from build123d import *

# Parameters (mm, degrees)
BOSS_EXTRUDE1_DEPTH = 6
BOSS_EXTRUDE2_DEPTH = 3
SKETCH3_W           = 15
SKETCH3_H           = 14.578547678
CUT_EXTRUDE1_DEPTH  = 3
CUT_EXTRUDE2_DEPTH  = 0.1
FILLET1_R           = 3
CHAMFER1_SIZE       = 0.528980942
CHAMFER1_SIZE_2     = 3


with BuildPart() as part:
    # Sketch1 → Boss-Extrude1 (new body)
    with BuildSketch(Plane(origin=(0, 0, 0), x_dir=(1, 0, 0), z_dir=(0, 1, 0))):
        with BuildLine():
            Line((22.5, -167.846096908), (22.5, -150.861139315))
            ThreePointArc((22.5, -150.861139315), (0, -153.564064606), (-22.5, -150.861139315))
            Line((-22.5, -150.861139315), (-22.5, -167.846096908))
            Line((-22.5, -167.846096908), (22.5, -167.846096908))
        make_face()
        with BuildLine():
            Line((-17.5, -154.846096908), (-17.5, -160.846096908))
            ThreePointArc((-17.5, -160.846096908), (-15.75, -162.596096908), (-14, -160.846096908))
            Line((-14, -160.846096908), (-14, -154.846096908))
            ThreePointArc((-14, -154.846096908), (-15.75, -153.096096908), (-17.5, -154.846096908))
        make_face(mode=Mode.SUBTRACT)
        with BuildLine():
            Line((14, -154.846096908), (14, -160.846096908))
            ThreePointArc((14, -160.846096908), (15.75, -162.596096908), (17.5, -160.846096908))
            Line((17.5, -160.846096908), (17.5, -154.846096908))
            ThreePointArc((17.5, -154.846096908), (15.75, -153.096096908), (14, -154.846096908))
        make_face(mode=Mode.SUBTRACT)
    extrude(amount=BOSS_EXTRUDE1_DEPTH)

    # Sketch2 → Boss-Extrude2 (add)
    with BuildSketch(Plane(origin=(0, 0, 0), x_dir=(1, 0, 0), z_dir=(0, 1, 0))):
        with BuildLine():
            Line((-22.5, -167.846096908), (22.5, -167.846096908))
            Line((22.5, -167.846096908), (22.5, -150.861139315))
            Line((22.5, -150.861139315), (10.691043752, -131.369092702))
            ThreePointArc((10.691043752, -131.369092702), (0, -125.346096908), (-10.691043752, -131.369092702))
            Line((-10.691043752, -131.369092702), (-22.5, -150.861139315))
            Line((-22.5, -150.861139315), (-22.5, -167.846096908))
        make_face()
        with BuildLine():
            Line((-17.5, -154.846096908), (-17.5, -160.846096908))
            ThreePointArc((-17.5, -160.846096908), (-15.75, -162.596096908), (-14, -160.846096908))
            Line((-14, -160.846096908), (-14, -154.846096908))
            ThreePointArc((-14, -154.846096908), (-15.75, -153.096096908), (-17.5, -154.846096908))
        make_face(mode=Mode.SUBTRACT)
        with BuildLine():
            Line((14, -154.846096908), (14, -160.846096908))
            ThreePointArc((14, -160.846096908), (15.75, -162.596096908), (17.5, -160.846096908))
            Line((17.5, -160.846096908), (17.5, -154.846096908))
            ThreePointArc((17.5, -154.846096908), (15.75, -153.096096908), (14, -154.846096908))
        make_face(mode=Mode.SUBTRACT)
    extrude(amount=BOSS_EXTRUDE2_DEPTH)

    # Sketch3 → Cut-Extrude1 (cut)
    with BuildSketch(Plane(origin=(0, 6, 0), x_dir=(1, 0, 0), z_dir=(0, 1, 0))):
        with Locations((0, -160.556823069)):
            Rectangle(SKETCH3_W, SKETCH3_H)
    extrude(amount=-CUT_EXTRUDE1_DEPTH, mode=Mode.SUBTRACT)

    # Sketch4 → Cut-Extrude2 (cut)
    with BuildSketch(Plane(origin=(0, 3, 0), x_dir=(1, 0, 0), z_dir=(0, 1, 0))):
        with BuildLine():
            Line((-4.25, -146.342419642), (-4.25, -167.846096908))
            Line((-4.25, -167.846096908), (4.25, -167.846096908))
            Line((4.25, -167.846096908), (4.25, -146.342419642))
            ThreePointArc((4.25, -146.342419642), (0, -128.346096908), (-4.25, -146.342419642))
        make_face()
    extrude(amount=-CUT_EXTRUDE2_DEPTH, mode=Mode.SUBTRACT)

    # Fillet1
    # the kernel refuses this fillet: 3 mm, written as the material it takes off along each edge
    with BuildSketch(Plane(origin=(-4.25, 2.9, 167.846096908), x_dir=(0, -1, 0), z_dir=(1, 0, 0))) as fillet1_piece_1:
        with BuildLine():
            CenterArc((FILLET1_R, FILLET1_R), FILLET1_R, 180, 90)
            Line((0, FILLET1_R), (0, 0))
            Line((0, 0), (FILLET1_R, 0))
        make_face()
    extrude(amount=8.5, mode=Mode.SUBTRACT)

    # Chamfer1
    # the kernel refuses this chamfer: 3, 0.528980942 mm, written as the material it takes off along each edge
    with BuildSketch(Plane(origin=(26.539379212, 3, 157.528601387), x_dir=(0.1797282148286355, -0.9776715712462603, -0.10888557099717337), z_dir=(-0.5181603365296565, 0, -0.8552835001608959))) as chamfer1_piece_1_section:
        Polygon((CHAMFER1_SIZE * 0.977671571478, CHAMFER1_SIZE * 0.210138760817), (-CHAMFER1_SIZE_2 * 0.210138760767, CHAMFER1_SIZE_2 * 0.977671571246), (0, 0), align=None)
    chamfer1_piece_1 = extrude(amount=30.585774986, mode=Mode.PRIVATE)
    chamfer1_piece_1 = chamfer1_piece_1 & Plane(origin=(0, 2.81678549, 58.564064606), x_dir=(0.23684210526315766, 0, 0.9715481548407755), z_dir=(0, -1, 0)) * Cylinder(95, 73, mode=Mode.PRIVATE)
    add(chamfer1_piece_1, mode=Mode.SUBTRACT)
    with BuildSketch(Plane(origin=(0, 3, 137.846096908), x_dir=(0.8552835001609747, 0, -0.5181603365295261), z_dir=(0.5181603365295261, 0, 0.8552835001609747))) as chamfer1_piece_2:
        Polygon((12.5, -CHAMFER1_SIZE), (12.5 - CHAMFER1_SIZE_2, 0), (12.5, 0), align=None)
    revolve(axis=Axis((0, 3, 137.846096908), (0, 1, 0)), revolution_arc=117.582137566, mode=Mode.SUBTRACT)
    with BuildSketch(Plane(origin=(-10.691043752, 3, 131.369092702), x_dir=(0.8552644030796279, 0.0066825316561016845, 0.5181487668570801), z_dir=(-0.5181603365296562, 0, 0.855283500160896))) as chamfer1_piece_3_section:
        Polygon((CHAMFER1_SIZE_2 * 0.999977671636, -CHAMFER1_SIZE_2 * 0.0066825316561), (-CHAMFER1_SIZE * 0.00668253165769, -CHAMFER1_SIZE * 0.999977671873), (0, 0), align=None)
    chamfer1_piece_3 = extrude(amount=30.585774986, mode=Mode.PRIVATE)
    chamfer1_piece_3 = chamfer1_piece_3 & Plane(origin=(0, 2.847950314, 58.564064606), x_dir=(0.23684210526315766, 0, 0.9715481548407755), z_dir=(0, -1, 0)) * Cylinder(95, 74, mode=Mode.PRIVATE)
    add(chamfer1_piece_3, mode=Mode.SUBTRACT)


solid = part.part
Verification items for the finished model (mm, model axes). A direction names the side the tool comes from. Give positions to 0.01 mm unless a question says otherwise; leave off trailing zeros. Write each loop counter-clockwise with the first axis right and the second up, starting at its lowest first coordinate (ties: lowest second). Pieces come first, ordered by that corner, then holes.
(1) Gauge pin test, flat ends, axial feed: pin 1 (1.5 mm diameter, centred on y = 2.5, z = 131, fed in from -X); pin 2 (8 mm diameter, centred on x = -3, z = 149.5, fed in from +Y); pin 3 (1 mm diameter, centred on y = 2, z = 137, fed in from -X). Record the tip position at first contact, or that the pin passes through.
(2) Cross-section at D-D (y = 0.9). Enter the section's corners in (x, z), plus the area to 3 significant figures.
(3) Material ranges on line 1 (X direction, y = 1.7, z = 160.5); line 2 (Y direction, x = 2, z = 144.5); line 3 (X direction, y = 4.65, z = 164), recorded low to high.
(4) Cross-section at B-B (z = 159). Enter the section's corners in (x, y).
(5) Cross-section at A-A (y = 4.3). Enter the section's corners in (x, z).
(6) Cross-section at C-C (x = -15.75). Enter the section's corners in (y, z).
(7) Access from +Z, -Z, +X, -X, +Y, -Y to the whole of each face (thin tool, end or side, straight path). Record for faces 5 (the face through (0, 0, 151)), 6 (the face through (0, 2.9, 142)), 7 (the face through (7.5, 5, 161)), 8 (the face through (-17.5, 3, 158)), 9 (the face through (-13, 6, 161)).
(8) Mould release check, pull along Z, two halves, no side actions. Record for faces 1 (the face through (-15.21, 2.74, 141.77)), 2 (the face through (10, 3, 152)), 3 (the face through (17.5, 3, 158)), 4 (the face through (-0.059, 2.079, 166.908)): +Z half, -Z half, draft (parallel to the pull), parting line (faces both ways), or undercut.
Worked out:
1. pin 1: stops at x = -10.92
1. pin 2: stops at y = 3
1. pin 3: stops at x = -14.41
2. outline: (-22.5, 150.86) - (-10.69, 131.37) arc R12.5 ccw to (10.69, 131.37) - (22.5, 150.86) - (22.5, 167.85) - (4.25, 167.85) - (4.25, 167.67) - (-4.25, 167.67) - (-4.25, 167.85) - (-22.5, 167.85) - close; hole (-17.5, 154.85) arc R1.75 ccw to (-14, 154.85) - (-14, 160.85) arc R1.75 ccw to (-17.5, 160.85) - close; hole (14, 154.85) arc R1.75 ccw to (17.5, 154.85) - (17.5, 160.85) arc R1.75 ccw to (14, 160.85) - close
2. area: 1,440 mm2
3. line 1: x = -22.5 to -17.5, -14 to 14, 17.5 to 22.5
3. line 2: y = 0 to 2.9
3. line 3: x = -22.5 to -7.5, 7.5 to 22.5
4. outline: (-22.5, 0) - (-17.5, 0) - (-17.5, 6) - (-22.5, 6) - close; (-14, 0) - (14, 0) - (14, 6) - (7.5, 6) - (7.5, 3) - (4.25, 3) - (4.25, 2.9) - (-4.25, 2.9) - (-4.25, 3) - (-7.5, 3) - (-7.5, 6) - (-14, 6) - close; (17.5, 0) - (22.5, 0) - (22.5, 6) - (17.5, 6) - close
5. outline: (-22.5, 150.86) arc R95 cw to (-7.5, 153.27) - (-7.5, 167.85) - (-22.5, 167.85) - close; (7.5, 153.27) arc R95 cw to (22.5, 150.86) - (22.5, 167.85) - (7.5, 167.85) - close; hole (-17.5, 154.85) arc R1.75 ccw to (-14, 154.85) - (-14, 160.85) arc R1.75 ccw to (-17.5, 160.85) - close; hole (14, 154.85) arc R1.75 ccw to (17.5, 154.85) - (17.5, 160.85) arc R1.75 ccw to (14, 160.85) - close
6. outline: (0, 139.72) - (2.47, 139.72) - (3, 145.51) - (3, 152.25) - (6, 152.25) - (6, 153.1) - (0, 153.1) - close; (0, 162.6) - (6, 162.6) - (6, 167.85) - (0, 167.85) - close
7. face 5: +Z, -Z, +X, -X, -Y
7. face 6: +Y
7. face 7: +Z, -Z, +Y
7. face 8: +Y, -Y
7. face 9: +Z, -Z, +X, -X, +Y
8. face 1: -Z half
8. face 2: draft
8. face 3: undercut
8. face 4: +Z half
